```python
from build123d import *

# Parameters (mm, degrees)
SKETCH2_R                = 50.8
BOSS_EXTRUDE1_DEPTH      = 38.1
FUEL_D                   = 1.016
FUEL_DEPTH               = 25.4
FUELPATTERN_COUNT        = 6
FUELPATTERN_COPY_1_D     = 1.016
FUELPATTERN_COPY_1_DEPTH = 25.4
FUELPATTERN_COPY_2_D     = 1.016
FUELPATTERN_COPY_2_DEPTH = 25.4
FUELPATTERN_COPY_3_D     = 1.016
FUELPATTERN_COPY_3_DEPTH = 25.4
FUELPATTERN_COPY_4_D     = 1.016
FUELPATTERN_COPY_4_DEPTH = 25.4
FUELPATTERN_COPY_5_D     = 1.016
FUELPATTERN_COPY_5_DEPTH = 25.4
OX_D                     = 1.016
OX_DEPTH                 = 25.4
OXPATTERN_COUNT          = 4
OXPATTERN_COPY_1_D       = 1.016
OXPATTERN_COPY_1_DEPTH   = 25.4
OXPATTERN_COPY_2_D       = 1.016
OXPATTERN_COPY_2_DEPTH   = 25.4
OXPATTERN_COPY_3_D       = 1.016
OXPATTERN_COPY_3_DEPTH   = 25.4


with BuildPart() as part:
    # Sketch2 → Boss-Extrude1 (new body)
    with BuildSketch(Plane(origin=(0, 0, 0), x_dir=(1, 0, 0), z_dir=(0, 1, 0))):
        with Locations(Location((0, 0, 0), (0, 0, 90))):
            Circle(SKETCH2_R)
    extrude(amount=BOSS_EXTRUDE1_DEPTH)

    # Fuel
    with Locations(Plane(origin=(0, 0, 0), x_dir=(0, 0, -1), z_dir=(-0.7071067811865488, -0.7071067811865464, 0))):
        with Locations((-38.1, 4.490128061)):
            fuel = Hole(FUEL_D / 2, depth=FUEL_DEPTH)

    # FuelMirror: Fuel across plane
    add(fuel.mirror(Plane(origin=(0, 0, 0), x_dir=(0, 0, 1), z_dir=(1, 0, 0))), mode=Mode.SUBTRACT)

    # FuelPattern: Fuel ×6 about axis
    fuelpattern_axis = Axis((0, 0, 0), (0, 1, 0))
    for i in range(1, FUELPATTERN_COUNT):
        add(fuel.rotate(fuelpattern_axis, i * 360 / FUELPATTERN_COUNT), mode=Mode.SUBTRACT)

    # FuelPattern copy 1
    with Locations(Plane(origin=(0, 0, 0), x_dir=(-0.8660254037844386, 0, -0.5000000000000001), z_dir=(0.35355339059327445, -0.7071067811865464, -0.6123724356957956))):
        with Locations((-38.1, -4.490128061)):
            Hole(FUELPATTERN_COPY_1_D / 2, depth=FUELPATTERN_COPY_1_DEPTH)

    # FuelPattern copy 2
    with Locations(Plane(origin=(0, 0, 0), x_dir=(-0.8660254037844387, 0, 0.4999999999999998), z_dir=(-0.35355339059327423, -0.7071067811865464, -0.6123724356957957))):
        with Locations((-38.1, -4.490128061)):
            Hole(FUELPATTERN_COPY_2_D / 2, depth=FUELPATTERN_COPY_2_DEPTH)

    # FuelPattern copy 3
    with Locations(Plane(origin=(0, 0, 0), x_dir=(0, 0, 1), z_dir=(-0.7071067811865488, -0.7071067811865464, 0))):
        with Locations((-38.1, -4.490128061)):
            Hole(FUELPATTERN_COPY_3_D / 2, depth=FUELPATTERN_COPY_3_DEPTH)

    # FuelPattern copy 4
    with Locations(Plane(origin=(0, 0, 0), x_dir=(0.8660254037844384, 0, 0.5000000000000004), z_dir=(-0.35355339059327473, -0.7071067811865464, 0.6123724356957955))):
        with Locations((-38.1, -4.490128061)):
            Hole(FUELPATTERN_COPY_4_D / 2, depth=FUELPATTERN_COPY_4_DEPTH)

    # FuelPattern copy 5
    with Locations(Plane(origin=(0, 0, 0), x_dir=(0.8660254037844386, 0, -0.5000000000000001), z_dir=(0.35355339059327445, -0.7071067811865464, 0.6123724356957956))):
        with Locations((-38.1, -4.490128061)):
            Hole(FUELPATTERN_COPY_5_D / 2, depth=FUELPATTERN_COPY_5_DEPTH)

    # Ox
    with Locations(Plane(origin=(0, 0, 0), x_dir=(0, 0, -1), z_dir=(-0.7071067811865488, -0.7071067811865464, 0))):
        with Locations((-12.7, 4.490128061)):
            ox = Hole(OX_D / 2, depth=OX_DEPTH)

    # OxMirror: Ox across plane
    add(ox.mirror(Plane(origin=(0, 0, 0), x_dir=(0, 0, 1), z_dir=(1, 0, 0))), mode=Mode.SUBTRACT)

    # OxPattern: Ox ×4 about axis
    oxpattern_axis = Axis((0, 0, 0), (0, 1, 0))
    for i in range(1, OXPATTERN_COUNT):
        add(ox.rotate(oxpattern_axis, i * 360 / OXPATTERN_COUNT), mode=Mode.SUBTRACT)

    # OxPattern copy 1
    with Locations(Plane(origin=(0, 0, 0), x_dir=(-1, 0, 0), z_dir=(0, -0.7071067811865464, -0.7071067811865488))):
        with Locations((-12.7, -4.490128061)):
            Hole(OXPATTERN_COPY_1_D / 2, depth=OXPATTERN_COPY_1_DEPTH)

    # OxPattern copy 2
    with Locations(Plane(origin=(0, 0, 0), x_dir=(0, 0, 1), z_dir=(-0.7071067811865488, -0.7071067811865464, 0))):
        with Locations((-12.7, -4.490128061)):
            Hole(OXPATTERN_COPY_2_D / 2, depth=OXPATTERN_COPY_2_DEPTH)

    # OxPattern copy 3
    with Locations(Plane(origin=(0, 0, 0), x_dir=(1, 0, 0), z_dir=(0, -0.7071067811865464, 0.7071067811865488))):
        with Locations((-12.7, -4.490128061)):
            Hole(OXPATTERN_COPY_3_D / 2, depth=OXPATTERN_COPY_3_DEPTH)


solid = part.part
```
For this review, take the finished solid that the model builds, in its own axes (mm). Round coordinates to 2 decimals unless told otherwise and drop trailing zeros. Loops run counter-clockwise (first coordinate to the right, second up) from the corner with the lowest first, then second, coordinate; pieces in that order, holes last.
(1) We need section A-A (y = 32). Give the boundary of the cut face in (x, z), plus the area to 3 significant figures.
Returned:
outline: circle Ø101.6 at (0, 0)
area: 8,110 mm2
(2) Wall thickness on line 1 along Z through (x, y) = (-26, 8); line 2 along X through (y, z) = (14.5, -21); line 3 along X through (y, z) = (11.5, -1.5): over which ranges is each line inside the solid? List them lowest first.
Returned:
line 1: z = -43.64 to -32.02, -30.81 to 30.81, 32.02 to 43.64
line 2: x = -46.26 to -13.2, -12.2 to 12.2, 13.2 to 46.26
line 3: x = -50.78 to 50.78
(3) We need section B-B (x = -41). State how many separate pieces and enclosed holes the cut face has, plus the area to 3 significant figures.
Returned:
separate pieces: 1
enclosed holes: 2
area: 2,280 mm2
(4) Clearance check with flat-ended pins moving along their axes: P1, Ø4, axis at x = 21, y = 18, coming from the +Z side; P2, Ø2, axis at y = 10.5, z = -3.5, coming from the -X side; P3, Ø3, axis at x = 18.5, y = 14, coming from the -Z side. State where each tip first meets the part, or that it passes through.
Returned:
P1: stops at z = 47.11
P2: stops at x = -50.74
P3: stops at z = -47.87
(5) Mouldability with a two-part tool opening along X and no side actions: class faces 1 (the flat face through (-1, 0, 1)), 2 (the cylindrical face through (40.286, 7.176, 7.392)) as released by +X, released by -X, zero draft, split by the parting line, or undercut.
Returned:
face 1: zero draft
face 2: undercut
